Geometry: final body of the model. Coordinates: model frame, mm. Coordinates: 2 decimals unless noted, no trailing zeros. Write each loop counter-clockwise with the first axis right and the second up, starting at its lowest first coordinate (ties: lowest second). Pieces come first, ordered by that corner, then holes. Notation, with made-up numbers: (-35, 72) -> (-8, 72) arc R15 ccw to (-8, 93) -> close; hole circle Ø7 at (-36.5, 83.5). An arc over 180 degrees is marked (long way). One line per item, written item: value.
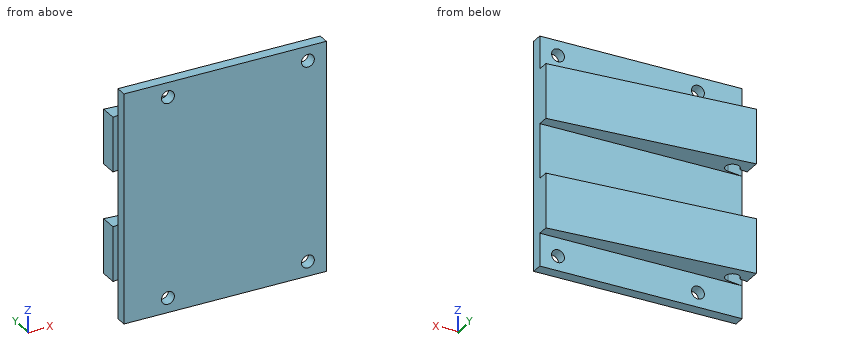
```python
from build123d import *

# Parameters (mm, degrees)
BOSS_EXTRUDE1_DEPTH     = 63
CUT_EXTRUDE1_START      = 24
CUT_EXTRUDE1_DEPTH      = 15
CUT_EXTRUDE1_2_DEPTH    = 9
CUT_EXTRUDE1_START_2    = 54
CUT_EXTRUDE1_3_DEPTH    = 9
CUT_EXTRUDE2_DEPTH      = 78.723870207
CUT_EXTRUDE2_DEPTH_BACK = 78.723870207
SKETCH3_R               = 1.9
SKETCH4_R               = 1.75
CUT_EXTRUDE3_DEPTH      = 84.891904797
CUT_EXTRUDE4_DEPTH      = 78.723870207


# Read off the part's stored shape, not the designer's step: Cut-Extrude1
with BuildPart() as part:
    # Sketch1 → Boss-Extrude1 (new body)
    with BuildSketch(Plane.XY):
        Polygon((0, 0), (55, -0.860341408), (55, 5.139658592), (0, 10), align=None)
    extrude(amount=BOSS_EXTRUDE1_DEPTH)

    # Cut-Extrude1 outline → Cut-Extrude1 (cut)
    with BuildSketch(Plane.XY.offset(CUT_EXTRUDE1_START)):
        Polygon((0, 10), (0, 3), (55, 2.139658592), (55, 5.139658592), align=None)
    extrude(amount=CUT_EXTRUDE1_DEPTH, mode=Mode.SUBTRACT)

    # Cut-Extrude1 2 outline → Cut-Extrude1 2 (cut)
    with BuildSketch(Plane.XY):
        Polygon((0, 10), (0, 3), (55, 2.139658592), (55, 5.139658592), align=None)
    extrude(amount=CUT_EXTRUDE1_2_DEPTH, mode=Mode.SUBTRACT)

    # Cut-Extrude1 3 outline → Cut-Extrude1 3 (cut)
    with BuildSketch(Plane.XY.offset(CUT_EXTRUDE1_START_2)):
        Polygon((0, 10), (0, 3), (55, 2.139658592), (55, 5.139658592), align=None)
    extrude(amount=CUT_EXTRUDE1_3_DEPTH, mode=Mode.SUBTRACT)

    # Sketch3 → Cut-Extrude2 (cut, two sides: drawn at the far end of the back side and taken through both)
    with BuildSketch(Plane(origin=(0, 0, 9), x_dir=(-1, 0, 0), z_dir=(0, 0, -1)).offset(-CUT_EXTRUDE2_DEPTH_BACK)):
        with Locations(Location((-4, 5.438102572, 0), (0, 0, 90))):
            Circle(SKETCH3_R)
    extrude(amount=CUT_EXTRUDE2_DEPTH + CUT_EXTRUDE2_DEPTH_BACK, mode=Mode.SUBTRACT)

    # Sketch4 → Cut-Extrude3 (cut, through all)
    with BuildSketch(Plane(origin=(0.046916233, 2.999266109, 0), x_dir=(0.9998776774332501, -0.01564065761691552, 0), z_dir=(0.01564065761691552, 0.9998776774332501, 0))):
        with Locations(Location((11.953078027, -59, 0), (0, 0, 180))):
            Circle(SKETCH4_R)
        with Locations(Location((50, -59, 0), (0, 0, 180))):
            Circle(SKETCH4_R)
        with Locations(Location((50, -4, 0), (0, 0, 180))):
            Circle(SKETCH4_R)
        with Locations(Location((11.953078027, -4, 0), (0, 0, 180))):
            Circle(SKETCH4_R)
    extrude(amount=-CUT_EXTRUDE3_DEPTH, mode=Mode.SUBTRACT)

    # Sketch6 → Cut-Extrude4 (cut, through all)
    with BuildSketch(Plane.XY.offset(54)):
        Polygon((2.117680715, 5.69670286), (0, 5.420349449), (0, 3), (4.245861834, 3.554077106), align=None)
    extrude(amount=-CUT_EXTRUDE4_DEPTH, mode=Mode.SUBTRACT)


solid = part.part
```
(1) Section D-D (x = 49). State how many separate pieces and enclosed holes the cut face has, then the cut area to 3 significant figures.
Responses:
separate pieces: 3
enclosed holes: 0
area: 275 mm2
(2) Line query: line 1 (Z direction, x = 10.5, y = 3.25); line 2 (Z direction, x = 49, y = 2); line 3 (Y direction, x = 5, z = 17.5). Output: solid intervals per line, ascending. Write a range as [from, to].
Responses:
line 1: z = [9, 24], [39, 54]
line 2: z = [0, 2.59], [5.41, 57.59], [60.41, 63]
line 3: y = [-0.08, 3.82], [7.05, 9.56]
(3) Section B-B (y = 9.25). Return the cut outline in (x, z), then the cut area to 3 significant figures.
Responses:
outline: (0, 9) -> (8.49, 9) -> (8.49, 24) -> (0, 24) -> close; (0, 39) -> (8.49, 39) -> (8.49, 54) -> (0, 54) -> close
area: 255 mm2
(4) Section C-C (x = 28.5). Return the cut outline in (y, z), then the cut area to 3 significant figures.
Responses:
outline: (-0.45, 0) -> (2.55, 0) -> (2.55, 9) -> (7.48, 9) -> (7.48, 24) -> (2.55, 24) -> (2.55, 39) -> (7.48, 39) -> (7.48, 54) -> (2.55, 54) -> (2.55, 63) -> (-0.45, 63) -> close
area: 337 mm2
(5) First-contact query: pin 1 (2.5 mm diameter, centred on x = 32, y = 5.5, fed in from -Z); pin 2 (12 mm diameter, centred on x = 27, z = 29.5, fed in from -Y); pin 3 (4 mm diameter, centred on x = 22.5, z = 48.5, fed in from +Y). Flat tips, straight axial feed; report the tip coordinate or a pass-through.
Responses:
pin 1: stops at z = 9
pin 2: stops at y = -0.52
pin 3: stops at y = 8.19
(6) Section A-A (z = 41.5). Return the cut outline in (x, y).
Responses:
outline: (0, 0) -> (55, -0.86) -> (55, 5.14) -> (0, 10) -> (0, 5.42) -> (2.12, 5.7) arc R1.9 cw (long way) to (4.25, 3.55) -> (0, 3) -> close
